Can you work these out from the drawing? Everything is in mm from the part's minimum corner. A direction names the side the tool comes from. Give positions to 0.01 mm unless a question says otherwise; leave off trailing zeros. Write each loop counter-clockwise with the first axis right and the second up, starting at its lowest first coordinate (ties: lowest second). Pieces come first, ordered by that corner, then holes. Notation, with made-up numbers: (-29, 86.5) - (24, 86.5) arc R22 cw to (24, 116.5) - close; hole circle Ø4 at (35.25, 23.5). An arc over 180 degrees is marked (long way). Use a Markdown table: item, result.
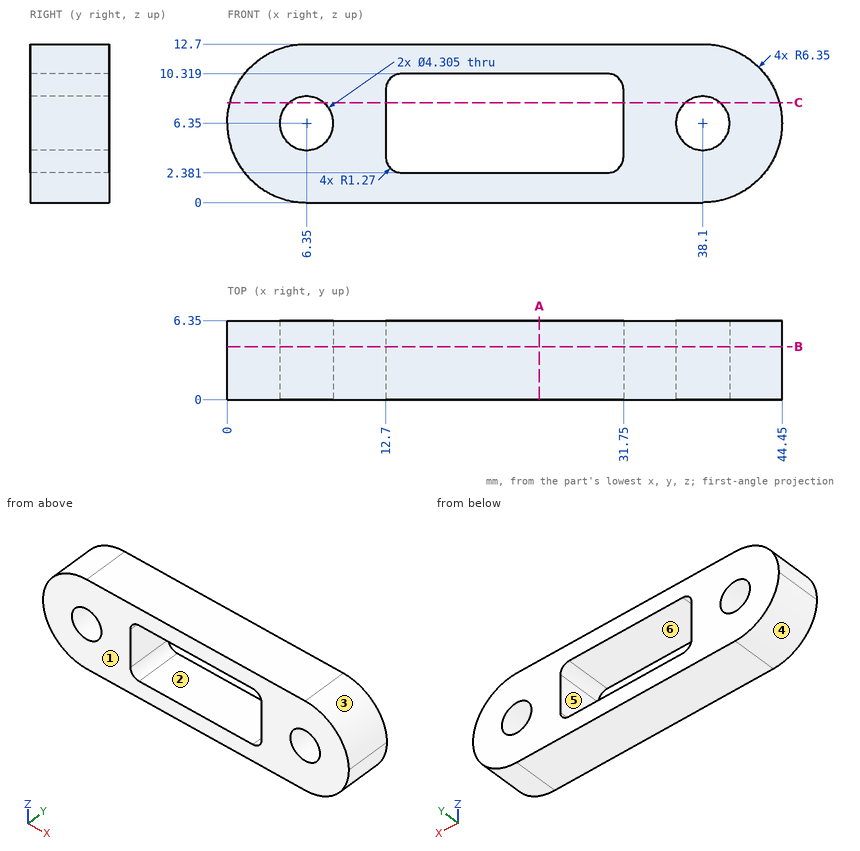
Item 1: I need wall thicknesses on line 1 along Z through (x, y) = (38, 6); line 2 along Z through (x, y) = (18, 1.75); line 3 along X through (y, z) = (3.75, 9.5). Which ranges of each line are inside material? Lowest first, please. Write a range as [from, to].
Values:
| item | result |
|---|---|
| line 1 | z = [0, 4.2], [8.5, 12.7] |
| line 2 | z = [0, 2.38], [10.32, 12.7] |
| line 3 | x = [0.84, 12.78], [31.67, 43.61] |
Item 2: If we section it at C-C, the plane z = 8: Write out the boundary of the cut face in (x, y).
Values:
| item | result |
|---|---|
| outline | (0.22, 0) - (4.97, 0) - (4.97, 6.35) - (0.22, 6.35) - close; (7.73, 0) - (12.7, 0) - (12.7, 6.35) - (7.73, 6.35) - close; (31.75, 0) - (36.72, 0) - (36.72, 6.35) - (31.75, 6.35) - close; (39.48, 0) - (44.23, 0) - (44.23, 6.35) - (39.48, 6.35) - close |
Item 3: Will these pins go through, and if not, where does the flat tip stop? pin 1 Ø3 at (y, z) = (3, 8.5) entering from -X; pin 2 Ø3.5 at (x, z) = (38.1, 6.35) entering from -Y.
Values:
| item | result |
|---|---|
| pin 1 | stops at x = 0.03 |
| pin 2 | passes through |
Item 4: If we section it at B-B, the plane y = 4.25: Count the separate pieces of the cut face and the enclosed holes in it, plus the area to 3 significant figures.
Values:
| item | result |
|---|---|
| separate pieces | 1 |
| enclosed holes | 3 |
| area | 351 mm2 |
Item 5: Thinking about a two-plate mould opening in Z: for the marked faces 3, 4, 5 and 6, which applies, +Z half, -Z half, draft (parallel to the pull), parting line (faces both ways), or undercut?
Values:
| item | result |
|---|---|
| face 3 | +Z half |
| face 4 | -Z half |
| face 5 | undercut |
| face 6 | undercut |
Item 6: If we section it at A-A, the plane x = 25: Write out the boundary of the cut face in (y, z).
Values:
| item | result |
|---|---|
| outline | (0, 0) - (6.35, 0) - (6.35, 2.38) - (0, 2.38) - close; (0, 10.32) - (6.35, 10.32) - (6.35, 12.7) - (0, 12.7) - close |
Item 7: For the marked faces 1 and 2, which set-ups out of +Z, -Z, +X, -X, +Y, -Y let a thin tool reach every point of the face, with its end or its side?
Values:
| item | result |
|---|---|
| face 1 | +Z, -Z, +X, -X, -Y |
| face 2 | +Y, -Y |
